Check sheet for the modelled part. Datum: model origin and axes. Units: mm. Face numbers are marked on the shaded views. A direction names the side the tool comes from. Round coordinates to 2 decimals unless told otherwise and drop trailing zeros. Loops run counter-clockwise (first coordinate to the right, second up) from the corner with the lowest first, then second, coordinate; pieces in that order, holes last. Notation, with made-up numbers: (86.5, -7) - (123.5, -7) arc R25 cw to (123.5, 18) - close; hole circle Ø3 at (14, 53). An arc over 180 degrees is marked (long way). Put each result on its own line as item: value. Start each with the question number.
```python
from build123d import *

# Parameters (mm, degrees)
SKETCH1_W             = 60
SKETCH1_H             = 40
SKETCH1_R             = 2.5
SKETCH1_W_2           = 42
SKETCH1_H_2           = 22
BOSS_EXTRUDE1_DEPTH   = 3.175
SKETCH2_W             = 60
SKETCH2_H             = 50
BOSS_EXTRUDE2_DEPTH   = 5
F_4_0MM_DOWEL_HOLE1_D = 4


with BuildPart() as part:
    # Sketch1 → Boss-Extrude1 (new body)
    with BuildSketch(Plane(origin=(0, 0, 0), x_dir=(1, 0, 0), z_dir=(0, 1, 0))):
        Rectangle(SKETCH1_W, SKETCH1_H)
        with Locations(Location((25, 5, 0), (0, 0, 270))):
            Circle(SKETCH1_R, mode=Mode.SUBTRACT)
        with Locations(Location((-23.8, 5, 0), (0, 0, 270))):
            Circle(SKETCH1_R, mode=Mode.SUBTRACT)
        with Locations(Location((-23.8, -5, 0), (0, 0, 270))):
            Circle(SKETCH1_R, mode=Mode.SUBTRACT)
        with Locations(Location((25, -5, 0), (0, 0, 270))):
            Circle(SKETCH1_R, mode=Mode.SUBTRACT)
        with Locations((0.6, 0)):
            Rectangle(SKETCH1_W_2, SKETCH1_H_2, mode=Mode.SUBTRACT)
    extrude(amount=BOSS_EXTRUDE1_DEPTH)

    # Sketch2 → Boss-Extrude2 (add)
    with BuildSketch(Plane.XY.offset(20)):
        with Locations((0, 25)):
            Rectangle(SKETCH2_W, SKETCH2_H)
    extrude(amount=BOSS_EXTRUDE2_DEPTH)

    # Ø4.0mm Dowel Hole1 (through all)
    with Locations(Plane(origin=(0, 0, 20), x_dir=(-1, 0, 0), z_dir=(0, 0, -1))):
        with Locations((-24, 44), (24, 44), (-24, 22), (24, 22)):
            Hole(F_4_0MM_DOWEL_HOLE1_D / 2)


solid = part.part
```
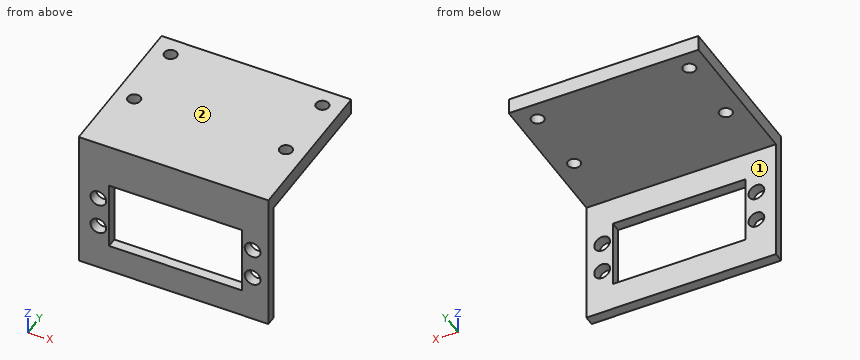
Q1. Cross-section at B-B on y = 22. Enter the section's corners in (x, z), and give its area (3 significant figures).
Q2. Cross-section at A-A on x = -13.5. Enter the section's corners in (y, z) (3 decimals).
Q3. Set-up check for the marked faces 1 and 2: record each of +Z, -Z, +X, -X, +Y, -Y from which the full face is reachable in a straight line by a thin tool's end or side.
Q4. Material ranges on line 1 (Y direction, x = -24, z = 21.5); line 2 (Y direction, x = -23, z = 0) (3 decimals); line 3 (Z direction, x = -1.5, y = 15), recorded low to high. Write a range as from..to.
Q5. Cross-section at D-D on x = 24. Enter the section's corners in (y, z) (3 decimals), and give its area (3 significant figures).
Q6. Depth check by flat-ended pin: pin 1 Ø5 at (x, y) = (24, 22) entering from -Z; pin 2 Ø6.5 at (x, z) = (-23.8, -5) entering from +Y (3 decimals); pin 3 Ø4 at (x, z) = (25, -5) entering from +Y. Enter the tip coordinate at first touch or a pass-through.
Q7. Cross-section at C-C on z = 3.5. Enter the section's corners in (x, y) (3 decimals).
Answer list:
1. outline: (-30, 20) - (-26, 20) - (-26, 25) - (-30, 25) - close; (-22, 20) - (22, 20) - (22, 25) - (-22, 25) - close; (26, 20) - (30, 20) - (30, 25) - (26, 25) - close
1. area: 260 mm2
2. outline: (0, -20) - (3.175, -20) - (3.175, -11) - (0, -11) - close; (0, 11) - (3.175, 11) - (3.175, 20) - (50, 20) - (50, 25) - (0, 25) - close
3. face 1: -Z, +X, -X, +Y
3. face 2: +Z, +X, -X, +Y, -Y
4. line 1: y = 0..20, 24..42, 46..50
4. line 2: y = 0..3.175
4. line 3: z = 20..25
5. outline: (0, -20) - (3.175, -20) - (3.175, -7.291) - (0, -7.291) - close; (0, -2.709) - (3.175, -2.709) - (3.175, 2.709) - (0, 2.709) - close; (0, 7.291) - (3.175, 7.291) - (3.175, 20) - (20, 20) - (20, 25) - (0, 25) - close; (24, 20) - (42, 20) - (42, 25) - (24, 25) - close; (46, 20) - (50, 20) - (50, 25) - (46, 25) - close
5. area: 308 mm2
6. pin 1: stops at z = 20
6. pin 2: stops at y = 3.175
6. pin 3: passes through
7. outline: (-30, 0) - (-25.8, 0) - (-25.8, 3.175) - (-30, 3.175) - close; (-21.8, 0) - (-20.4, 0) - (-20.4, 3.175) - (-21.8, 3.175) - close; (21.6, 0) - (23, 0) - (23, 3.175) - (21.6, 3.175) - close; (27, 0) - (30, 0) - (30, 3.175) - (27, 3.175) - close
